Can you work these out from the model? Positions are in its coordinate system, mm. A direction names the side the tool comes from. Give positions to 0.01 mm unless a question says otherwise; leave off trailing zeros. Loops run counter-clockwise (first coordinate to the right, second up) from the corner with the lowest first, then second, coordinate; pieces in that order, holes last. Notation, with made-up numbers: M 0,68.5 L 12,68.5 A12 cw 12,91.5 Z; hole C 0,47 d5. An arc over 180 degrees is marked long. One line per item, written item: value. Start each with the question number.
Autodesk Inventor part; units mm, degrees
ref_plane "YZ Plane" through (0, 0, 0) normal (1, 0, 0) x (0, 1, 0)
ref_plane "XZ Plane" through (0, 0, 0) normal (0, 1, 0) x (-1, 0, 0)
ref_plane "XY Plane" through (0, 0, 0) normal (0, 0, 1) x (1, 0, 0)
sketch "Sketch1" plane through (0, 0, 0) normal (0, 0, 1) x (1, 0, 0)
  line L0 (0, 0) -> (1021.08, 0)
  line L1 (1021.08, 0) -> (1021.08, 50.8)
  line L2 (1021.08, 50.8) -> (0, 50.8)
  line L3 (0, 50.8) -> (0, 0)
  dimension "d0" = 1021.08
  dimension "d1" = 50.8
extrude "Plate1" add sketch "Sketch1" along normal blind 2.54
sketch "Sketch2" plane through (2.54, 0, 0) normal (-1, 0, 0) x (0, -1, 0)
  line L0 (-50.8, 0) -> (0, 0)
  line L1 (0, 0) -> (0, 27.94)
  line L2 (0, 27.94) -> (-50.8, 27.94)
  line L3 (-50.8, 27.94) -> (-50.8, 0)
edge flange "Flange1" height 27.94 angle 90 thickness 2.54 bend radius 2.54 thickness toward (-1, 0, 0) relief tear relief width 2.54 relief depth 1.27 corner gap 2.54 corner form 0 edges at (0, 25.4, 2.54) (1021.08, 25.4, 2.54) wall of the first edge with corners at (2.54, 50.8, 0) (2.54, 0, 0) (2.54, 0, 27.94) (2.54, 50.8, 27.94)
bend "Bend1"
corner "Corner1"
sketch "Sketch3" plane through (0, 0, 0) normal (0, 0, -1) x (-1, 0, 0)
  circle A0 centre (-317.326, 37.1303) radius 3.175
  circle A1 centre (-657.3374, 25.4) radius 3.175
  circle A2 centre (-363.7426, 25.4) radius 3.175
  point P0 (0, 0)
extrude "Extrusion1" cut sketch "Sketch3" against normal blind 25.4 contours A1 | A2
sketch "Sketch4" plane through (1021.08, 0, 27.94) normal (1, 0, 0) x (0, 0, -1)
  line L0 (0, 0) -> (22.86, 0)
  line L1 (22.86, 0) -> (22.86, 50.8)
  line L2 (22.86, 50.8) -> (0, 50.8)
  line L3 (0, 50.8) -> (0, 0)
  circle A0 centre (11.43, 38.1) radius 3.175
  circle A1 centre (11.43, 12.7) radius 3.175
  point P0 (27.94, 0)
  dimension "d15" = 6.35
  dimension "d16" = 6.35
extrude "Extrusion2" cut sketch "Sketch4" against normal blind 2.54 contours A0 | A1
sketch "Sketch5" plane through (0, 0, 27.94) normal (-1, 0, 0) x (0, 0, 1)
  line L0 (0, 50.8) -> (-22.86, 50.8)
  line L1 (-22.86, 50.8) -> (-22.86, 0)
  line L2 (-22.86, 0) -> (0, 0)
  line L3 (0, 0) -> (0, 50.8)
  circle A0 centre (-11.43, 38.1) radius 3.175
  circle A1 centre (-11.43, 12.7) radius 3.175
  circle A2 centre (-11.43, 12.7) radius 3.175
  circle A3 centre (-11.43, 38.1) radius 3.175
  point P0 (-27.94, 0)
extrude "Extrusion3" cut sketch "Sketch5" against normal blind 2.54 contours A0 | A1
equation "\"d3\" = BendReliefWidth"
equation "\"d4\" = BendReliefDepth"
equation "\"d5\" = MinimumRemnant"
equation "\"d6\" = BendRadius"
equation "\"d9\" = BendRadius"
equation "\"d10\" = CornerReliefSize"
equation "\"d11\" = GapSize"
equation "\"d12\" = JacobiRadiusSize"
equation "\"BendRadius\" = Thickness"
equation "\"BendReliefWidth\" = Thickness"
equation "\"BendReliefDepth\" = 0.5 * Thickness"
equation "\"CornerReliefSize\" = 4 * Thickness"
equation "\"MinimumRemnant\" = 2 * Thickness"
equation "\"TransitionRadius\" = BendRadius"
equation "\"JacobiRadiusSize\" = BendRadius"
equation "\"GapSize\" = Thickness"
equation "\"d2\" = BendRadius"
properties part number "bumper piece"
Q1. Which directions (+Z, -Z, +X, -X, +Y, -Y) give clear straight access to the entire face, cutting with the end or side of a thin tool? Please do faces 4 (the face through (2.54, 25, 16)), 5 (the face through (0, 25, 17)).
Q2. I need wall thicknesses on line 1 along Y through (x, z) = (1019.85, 16.51) (3 decimals); line 2 along X through (y, z) = (30.5, 24.25); line 3 along Z through (x, y) = (943, 38). Which ranges of each line are inside material? Lowest first, please.
Q3. If we mould it in two halves opening along X, with no side actions, what happens to faces 1 (the face through (503, 26, 2.54)), 2 (the face through (508, 50.8, 2)), 3 (the face through (1021.08, 26, 17))? For each: released by +X, released by -X, zero draft, split by the parting line, or undercut.
Q4. For P1, Ø5.5, axis at x = 363.74, y = 25.4, coming from the -Z side; P2, Ø15, axis at x = 538.5, y = 30, coming from the +Z side, each with a flat end and sliding along its axis, tell me the tip position at first contact or that it passes through.
Q5. If we section it at A-A, the plane x = 687.5: Write out the boundary of the cut face in (y, z), plus the area to 3 significant figures.
Response:
1. face 4: +Z, +Y, -Y
1. face 5: +Z, -Z, -X, +Y, -Y
2. line 1: 0 to 9.525, 15.875 to 34.925, 41.275 to 50.8
2. line 2: 0 to 2.54, 1018.54 to 1021.08
2. line 3: 0 to 2.54
3. face 1: undercut
3. face 2: zero draft
3. face 3: released by +X
4. P1: through
4. P2: z = 2.54
5. outline: M 0,0 L 50.8,0 L 50.8,2.54 L 0,2.54 Z
5. area: 129 mm^2
